The listing builds one solid part. Answer for the finished solid, in the listing's coordinates (mm). Round coordinates to 2 decimals unless told otherwise and drop trailing zeros. Write each loop counter-clockwise with the first axis right and the second up, starting at its lowest first coordinate (ties: lowest second). Pieces come first, ordered by that corner, then holes.
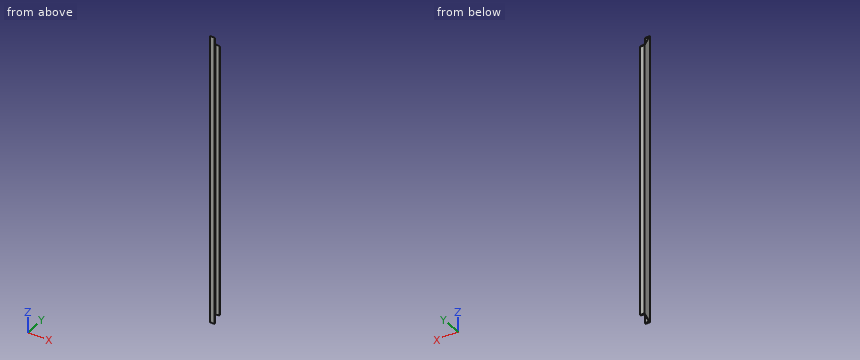
Autodesk Inventor part; units mm, degrees
ref_plane "Начальная плоскость" through (0, 0, -22.2222) normal (0, 0, 1) x (1, 0, 0)
ref_plane "Конечная плоскость" through (0, 0, 2954.7764) normal (0, 0, 1) x (1, 0, 0)
ref_plane "РабПлоскость4" through (91.07, 77.7029, 2742.9113) normal (0, 0.8742, 0.4856) x (1, 0, 0)
ref_plane "Начальная плоскость" through (0, 0, -22.2222) normal (0, 0, 1) x (1, 0, 0)
ref_plane "Конечная плоскость" through (0, 0, 2954.7764) normal (0, 0, 1) x (1, 0, 0)
sketch "Эскиз" plane through (0, 0, 0) normal (0, 0, 1) x (1, 0, 0)
  line L0 (-1.43, 0) -> (-1.43, 40)
  line L1 (-1.43, 40) -> (43.57, 40)
  line L2 (43.57, 40) -> (43.57, 38.1774)
  line L3 (39.9881, 34.1993) -> (11.2338, 31.1771)
  line L4 (4.07, 23.221) -> (4.07, 0)
  line L5 (4.07, 0) -> (-1.43, 0) construction
  line L6 (23.82, 40) -> (23.82, 32.5) construction
  line L7 (43.57, 34.5758) -> (43.57, 32.5) construction
  line L8 (43.57, 32.5) -> (23.82, 32.5) construction
  line L9 (0, 15) -> (0, -27) construction
  line L10 (-5.539, 0) -> (16.0067, 0) construction
  line L11 (-1.43, 0) -> (-1.43, -40)
  line L12 (-1.43, -40) -> (43.57, -40)
  line L13 (43.57, -40) -> (43.57, -38.1774)
  line L14 (39.9881, -34.1993) -> (11.2338, -31.1771)
  line L15 (4.07, -23.221) -> (4.07, 0)
  arc A0 (11.2338, 31.1771) -> (4.07, 23.221) centre (12.07, 23.221) ccw
  arc A1 (4.07, -23.221) -> (11.2338, -31.1771) centre (12.07, -23.221) ccw
  arc A2 (39.9881, 34.1993) -> (43.57, 38.1774) centre (39.57, 38.1774) ccw
  arc A3 (43.57, -38.1774) -> (39.9881, -34.1993) centre (39.57, -38.1774) ccw
  line L16 (0, 56) -> (0, -56) construction
  line L17 (-15.5135, 0) -> (54.308, 0) construction
  point P0 (4.07, 30.4242)
  point P1 (43.57, -34.5758)
  point P2 (4.07, -30.4242)
  point P3 (23.82, -40)
  point P4 (23.82, -32.5)
  dimension "d0" = 5.5
  dimension "d1" = 40
  dimension "d2" = 45
  dimension "d3" = 7.5
  dimension "d4" = 19.75
  dimension "d5" = 2.0758
  dimension "d23" = 8
  dimension "d24" = 4
  dimension "d25" = 1.43
extrude "Тело" add sketch "Эскиз" along normal up to surface (2976.9987 mm away) from surface at -22.2222
sketch "Sketch3" plane through (0, 0, 0) normal (0, 0, 1) x (1, 0, 0)
  line L0 (0, 0) -> (10, 0)
ref_plane "Work Plane3" through (0, 0, 0) normal (0, -1, 0) x (1, 0, 0)
sketch "Sketch4" plane through (0, 0, 0) normal (0, -1, 0) x (1, 0, 0)
  line L0 (-2, -22.2222) -> (12, -22.2222)
  line L1 (-2, 2954.7764) -> (12, 2954.7764)
  dimension "d29" = 2976.9987
ref_plane "РабПлоскость4" through (91.07, 77.7029, 2742.9113) normal (0, 0.8742, 0.4856) x (1, 0, 0)
split "Разделение1" plane through (91.07, 77.7029, 2742.9113) removes the side toward (0, 0.8742, 0.4856)
ref_plane "РабПлоскость5" through (91.07, 74.3034, 41.2796) normal (0, 0.4856, -0.8742) x (1, 0, 0)
split "Разделение2" plane through (91.07, 74.3034, 41.2796) removes the side toward (0, 0.4856, -0.8742)
equation "\"d0\" = G_T"
equation "\"d1\" = 0.5 * G_H"
equation "\"d2\" = G_W"
equation "\"d3\" = G_T1"
equation "\"d4\" = G_C"
equation "\"d23\" = G_IR"
equation "\"d24\" = G_ER"
equation "\"d25\" = ex"
equation "\"d6\" = G_L"
equation "\"G_W\" = 45"
equation "\"G_T\" = 5.5"
equation "\"G_T1\" = 7.5"
equation "\"G_NG\" = 0.105104"
equation "\"G_ER\" = 4"
equation "\"G_IR\" = 8"
equation "\"G_C\" = 19.75"
equation "\"G_L\" = d29"
equation "\"ex\" = 1.43"
equation "\"G_OFFSET_START\" = 22.22222"
equation "\"G_OFFSET_END\" = 72"
equation "\"d26\" = -G_OFFSET_START"
equation "\"d27\" = G_OFFSET_END + B_L"
equation "\"B_L\" = 2882.77644"
properties part number "ISO 657/11 - CH 80 x 8 - 2977" material "Сталь, мягкая"
1. Given pin 1 (23 mm diameter, centred on y = -6, z = 887, fed in from +X), flat-ended and moving along its own axis, determine where the tip first touches the part or whether it passes through.
Geometry says:
pin 1: stops at x = 4.07
2. Section C-C on y = -9.5 is taken. Determine the outline of the cut face in (x, z).
Geometry says:
outline: (-1.43, -5.27) - (4.07, -5.27) - (4.07, 2899.9) - (-1.43, 2899.9) - close
3. Section B-B on z = 2138 is taken. Determine the outline of the cut face in (x, y), plus the area to 3 significant figures.
Geometry says:
outline: (-1.43, -40) - (43.57, -40) - (43.57, -38.18) arc R4 ccw to (39.99, -34.2) - (11.23, -31.18) arc R8 cw to (4.07, -23.22) - (4.07, 23.22) arc R8 cw to (11.23, 31.18) - (39.99, 34.2) arc R4 ccw to (43.57, 38.18) - (43.57, 40) - (-1.43, 40) - close
area: 1,050 mm2
4. Straight lines are drawn through the part: line 1 along Y through (x, z) = (12, 1715.5); line 2 along Y through (x, z) = (37, 1188.5); line 3 along X through (y, z) = (-4.5, 2414.5). For each, find the intervals that lie inside material, in ascending order.
Geometry says:
line 1: y = -40 to -31.26, 31.26 to 40
line 2: y = -40 to -33.89, 33.89 to 40
line 3: x = -1.43 to 4.07
